Can you work these out from the model? Positions are in its coordinate system, mm. Face numbers are marked on the shaded views. A direction names the side the tool comes from. Give positions to 0.01 mm unless a question says otherwise; leave off trailing zeros. Loops run counter-clockwise (first coordinate to the right, second up) from the corner with the lowest first, then second, coordinate; pieces in that order, holes last. Notation, with made-up numbers: (76, -33) - (131, -33) arc R19 ccw to (131, -16) - close; hole circle Ø8 at (34.5, 13). An arc over 180 degrees is marked (long way). Answer in a Markdown table with one row per item.
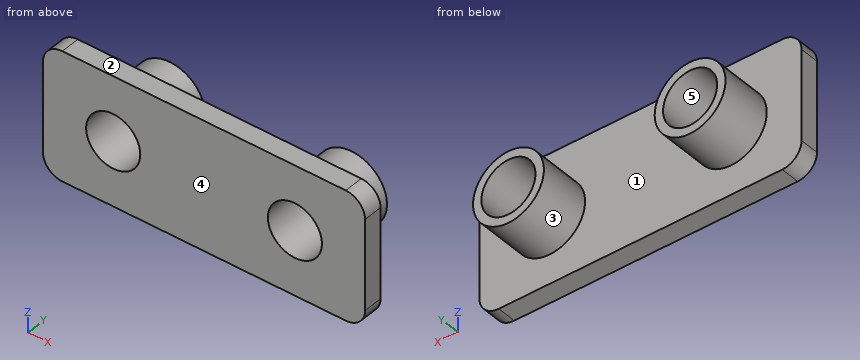
from build123d import *

# Parameters (mm, degrees)
SKETCH1_R           = 2.1
BOSS_EXTRUDE1_DEPTH = 1.5
SKETCH3_R           = 2.75
SKETCH3_R_2         = 2.1
BOSS_EXTRUDE2_DEPTH = 4


with BuildPart() as part:
    # Sketch1 → Boss-Extrude1 (new body)
    with BuildSketch(Plane(origin=(0, 0, 0), x_dir=(1, 0, 0), z_dir=(0, 1, 0))):
        with BuildLine():
            Line((-11, 5), (11, 5))
            ThreePointArc((11, 5), (12.060660172, 4.560660172), (12.5, 3.5))
            Line((12.5, 3.5), (12.5, -3.5))
            ThreePointArc((12.5, -3.5), (12.060660172, -4.560660172), (11, -5))
            Line((11, -5), (-11, -5))
            ThreePointArc((-11, -5), (-12.060660172, -4.560660172), (-12.5, -3.5))
            Line((-12.5, -3.5), (-12.5, 3.5))
            ThreePointArc((-12.5, 3.5), (-12.060660172, 4.560660172), (-11, 5))
        make_face()
        with Locations((-7.05, 0)):
            Circle(SKETCH1_R, mode=Mode.SUBTRACT)
        with Locations((7.05, 0)):
            Circle(SKETCH1_R, mode=Mode.SUBTRACT)
    extrude(amount=BOSS_EXTRUDE1_DEPTH)

    # Sketch3 → Boss-Extrude2 (add)
    with BuildSketch(Plane(origin=(0, 1.5, 0), x_dir=(1, 0, 0), z_dir=(0, 1, 0))):
        with Locations((-7.05, 0)):
            Circle(SKETCH3_R)
        with Locations((-7.05, 0)):
            Circle(SKETCH3_R_2, mode=Mode.SUBTRACT)
        with Locations((7.05, 0)):
            Circle(SKETCH3_R)
        with Locations((7.05, 0)):
            Circle(SKETCH3_R_2, mode=Mode.SUBTRACT)
    extrude(amount=BOSS_EXTRUDE2_DEPTH)


solid = part.part
Q1. Imagine slicing it at B-B, the plane x = 7.05. Write out the boundary of the cut face in (y, z), and give its area (3 significant figures).
Checked values:
| item | result |
|---|---|
| outline | (0, -5) - (1.5, -5) - (1.5, -2.75) - (5.5, -2.75) - (5.5, -2.1) - (0, -2.1) - close; (0, 2.1) - (5.5, 2.1) - (5.5, 2.75) - (1.5, 2.75) - (1.5, 5) - (0, 5) - close |
| area | 13.9 mm² |
Q2. On a 3-axis mill with a long thin cutter (end or side, diameter ignored), from which of +Z, -Z, +X, -X, +Y, -Y can I reach the whole of each face in a straight line? I mean the marked faces 1 and 2. Say none if no direction works.
Checked values:
| item | result |
|---|---|
| face 1 | +Y |
| face 2 | +Z, +X, -X, +Y, -Y |
Q3. Imagine slicing it at A-A, the plane y = 4.5. Write out the boundary of the cut face in (x, z), and give its area (3 significant figures).
Checked values:
| item | result |
|---|---|
| outline | circle Ø5.5 at (-7.05, 0); circle Ø5.5 at (7.05, 0); hole circle Ø4.2 at (-7.05, 0); hole circle Ø4.2 at (7.05, 0) |
| area | 19.8 mm² |
Q4. If we mould it in two halves opening along Z, with no side actions, what happens to the marked faces 3, 4 and 5? For each: released by +Z, released by -Z, zero draft, split by the parting line, or undercut.
Checked values:
| item | result |
|---|---|
| face 3 | split by the parting line |
| face 4 | zero draft |
| face 5 | undercut |
Q5. For pin 1 (2 mm diameter, centred on y = 3, z = -1.5, fed in from -X), with a flat end and sliding along its axis, tell me the tip position at first contact or that it passes through.
Checked values:
| item | result |
|---|---|
| pin 1 | stops at x = -9.75 |
Q6. Imagine slicing it at C-C, the plane z = 0. Write out the boundary of the cut face in (x, y).
Checked values:
| item | result |
|---|---|
| outline | (-12.5, 0) - (-9.15, 0) - (-9.15, 5.5) - (-9.8, 5.5) - (-9.8, 1.5) - (-12.5, 1.5) - close; (-4.95, 0) - (4.95, 0) - (4.95, 5.5) - (4.3, 5.5) - (4.3, 1.5) - (-4.3, 1.5) - (-4.3, 5.5) - (-4.95, 5.5) - close; (9.15, 0) - (12.5, 0) - (12.5, 1.5) - (9.8, 1.5) - (9.8, 5.5) - (9.15, 5.5) - close |
Q7. Imagine slicing it at D-D, the plane y = 0.7. Write out the boundary of the cut face in (x, z).
Checked values:
| item | result |
|---|---|
| outline | (-12.5, -3.5) arc R1.5 ccw to (-11, -5) - (11, -5) arc R1.5 ccw to (12.5, -3.5) - (12.5, 3.5) arc R1.5 ccw to (11, 5) - (-11, 5) arc R1.5 ccw to (-12.5, 3.5) - close; hole circle Ø4.2 at (-7.05, 0); hole circle Ø4.2 at (7.05, 0) |
Q8. If I drill on line 1 (Z direction, x = 7.05, y = 4.1); line 2 (X direction, y = 1.55, z = 1.5); line 3 (Y direction, x = 9.5, z = 4.75), over which ranges is the centre line in solid material (lowest first)? Write a range as [from, to].
Checked values:
| item | result |
|---|---|
| line 1 | z = [-2.75, -2.1], [2.1, 2.75] |
| line 2 | x = [-9.35, -8.52], [-5.58, -4.75], [4.75, 5.58], [8.52, 9.35] |
| line 3 | y = [0, 1.5] |
